Work out the finished part from the listing and answer in its coordinate system (mm). A direction names the side the tool comes from. Give positions to 0.01 mm unless a question says otherwise; leave off trailing zeros. Order: outer loops, then holes, each group sorted by start corner. A loop starts at its lowest first (then second) coordinate and runs counter-clockwise, first axis right, second up.
```python
from build123d import *

# Parameters (mm, degrees)
BOX_W     = 30
BOX_H     = 37
BOX_DEPTH = 13
PAD_DEPTH = 28


with BuildPart() as cube:
    # Box → Box (new body)
    with BuildSketch(Plane(origin=(-2, -32, 40), x_dir=(1, 0, 0), z_dir=(0, 0, 1))):
        with Locations((15, 18.5)):
            Rectangle(BOX_W, BOX_H)
    extrude(amount=BOX_DEPTH)


with BuildPart() as cut:
    # Sketch → Pad (new body)
    with BuildSketch(Plane.XZ):
        with BuildLine():
            Line((0, 0), (110, 0))
            Line((110, 0), (102, 25))
            ThreePointArc((102, 25), (99.099229, 29.583137), (94.332421, 32.171022))
            Line((94.332421, 32.171022), (45, 44.39))
            ThreePointArc((45, 44.39), (42.518536, 44.846937), (40, 45))
            Line((40, 45), (0, 45))
            Line((0, 45), (0, 0))
        make_face()
    extrude(amount=PAD_DEPTH)

    # Cut: cut Cube
    add(cube.part, mode=Mode.SUBTRACT)


solid = cut.part
```
1. The part is cut by section B-B (z = 19). Write down the section's boundary in (x, y), then the cut area to 3 significant figures.
Findings below:
outline: (0, -28) - (103.92, -28) - (103.92, 0) - (0, 0) - close
area: 2,910 mm2
2. The part is cut by section A-A (y = -6.5). Write down the section's boundary in (x, z).
Findings below:
outline: (0, 0) - (110, 0) - (102, 25) arc R10.77 ccw to (94.33, 32.17) - (45, 44.39) arc R20.8 ccw to (40, 45) - (28, 45) - (28, 40) - (0, 40) - close
3. Straight lines are drawn through the part: probe 1 along Z at (x, y) = (17.5, -18); probe 2 along Z at (x, y) = (56.5, -27); probe 3 along X at (y, z) = (-24, 15.5). For each, find the intervals that lie inside material, in ascending order.
Findings below:
probe 1: z = 0 to 40
probe 2: z = 0 to 41.54
probe 3: x = 0 to 105.04
4. Given P1, Ø5.5, axis at y = -17, z = 43.5, coming from the -X side; P2, Ø2, axis at y = -10, z = 10.5, coming from the +X side; P3, Ø10, axis at x = 81.5, y = -18, coming from the +Z side, each flat-ended and moving along its own axis, determine where each tip first touches the part or whether it passes through.
Findings below:
P1: stops at x = 28
P2: stops at x = 106.96
P3: stops at z = 36.59
5. Which of the six approach directions +Z, -Z, +X, -X, +Y, -Y give full straight-line access (tool end or side, diameter ignored) to faces 1 (the face through (14, -14, 40)), 2 (the face through (34, -14, 45))?
Findings below:
face 1: +Z, -X, +Y, -Y
face 2: +Z, +X, -X, +Y, -Y
6. The part is cut by section C-C (x = 90.5). Write down the section's boundary in (y, z), then the cut area to 3 significant figures.
Findings below:
outline: (-28, 0) - (0, 0) - (0, 33.12) - (-28, 33.12) - close
area: 927 mm2
